```python
from build123d import *

# Parameters (mm, degrees)
F1_DEPTH = 130
F3_D     = 7
F5_D     = 5
F7_DEPTH = 25


# Not quite as in the source:
# - a feature names something its author has since deleted; it is built from what else it names


with BuildPart() as f1:
    # F0 (on Front) → F1 (new body, symmetric)
    with BuildSketch(Plane.XZ):
        Polygon((0, 30), (0, 0), (3, 0), (3, 27), (30, 27), (30, 30), align=None)
    extrude(amount=F1_DEPTH, both=True)

    # F3 (through all)
    with Locations(Plane(origin=(0, 0, 0), x_dir=(0, -1, 0), z_dir=(-1, 0, 0))):
        with Locations((-31.5, 10), (31.5, 10)):
            Hole(F3_D / 2)

    # F5 (through all)
    with Locations(Plane.XY.offset(30)):
        with Locations((14.7187495604, 0), (14.7187495604, -100), (14.7187495604, 100), (14.7187495604, -120), (14.7187495604, 120)):
            Hole(F5_D / 2)

    # F6 (on face) → F7 (cut)
    with BuildSketch(Plane(origin=(0, 0, 0), x_dir=(0, -1, 0), z_dir=(-1, 0, 0))):
        Polygon((-85, 0), (-130, 25), (-130, 0), align=None)
        Polygon((130, 0), (130, 25), (85, 0), align=None)
    extrude(amount=-F7_DEPTH, mode=Mode.SUBTRACT)


solid = f1.part
```
Design review of the part built by this model. Coordinates are the model's own, in mm. A direction names the side the tool comes from. Coordinates: 2 decimals unless noted, no trailing zeros. Order: outer loops, then holes, each group sorted by start corner. A loop starts at its lowest first (then second) coordinate and runs counter-clockwise, first axis right, second up. Notation, with made-up numbers: (9, 87.25) -> (52, 87.25) arc R5 ccw to (52, 96.25) -> close; hole circle Ø10 at (11, -2). An arc over 180 degrees is marked (long way). One line per item, written item: value. Start each with the question number.
Q1. Insertion check: pin 1 Ø8 at (y, z) = (53.5, 5.5) entering from +X; pin 2 Ø6 at (x, y) = (22.5, 19.5) entering from -Z; pin 3 Ø10 at (x, z) = (4, 19.5) entering from -Y; pin 4 Ø1 at (y, z) = (103, 18.5) entering from -X. Each pin has a flat end and moves straight along its axis. Give the tip position at first contact, or say it passes through.
Q2. Take a section at C-C, the plane y = 0. State the section outline as (x, z) points, then the cut area to 3 significant figures.
Q3. Tool access review of faces 5 (the flat face through (19, -2, 27)), 6 (the flat face through (15, -130, 29)): name each direction out of +Z, -Z, +X, -X, +Y, -Y from which nothing blocks a thin tool from reaching the whole face with its end or side.
Q4. Take a section at D-D, the plane x = 21.25. State the section outline as (y, z) points, then the cut area to 3 significant figures.
Q5. For probe 1 along Z at (x, y) = (1.55, 31.5); probe 2 along X at (y, z) = (73, 20.5); probe 3 along Z at (x, y) = (22.75, -110), list the stretches that pass through material, from the lowest coordinate up.
Q6. Take a section at B-B, the plane z = 10. State the section outline as (x, y) points.
Q7. Mouldability with a two-part tool opening along Z and no side actions: class faces 1 (the flat face through (19, -2, 30)), 2 (the flat face through (1.479, -107.815, 12.675)), 3 (the flat face through (0, -2, 15)), 4 (the cylindrical face through (1.521, 33.115, 6.895)) as pulls with the +Z half, pulls with the -Z half, needs draft (parallel to the pull), parting line crosses it, or undercut.
Q8. Take a section at A-A, the plane y = 31.5. State the section outline as (x, z) points, then the cut area to 3 significant figures.
Values follow:
1. pin 1: stops at x = 3
1. pin 2: stops at z = 27
1. pin 3: stops at y = -128.92
1. pin 4: stops at x = 0
2. outline: (0, 0) -> (3, 0) -> (3, 27) -> (12.22, 27) -> (12.22, 30) -> (0, 30) -> close; (17.22, 27) -> (30, 27) -> (30, 30) -> (17.22, 30) -> close
2. area: 156 mm2
3. face 5: -Z, +X, +Y, -Y
3. face 6: +Z, -Z, +X, -X, -Y
4. outline: (-130, 27) -> (130, 27) -> (130, 30) -> (-130, 30) -> close
4. area: 780 mm2
5. probe 1: z = 0 to 6.5, 13.5 to 30
5. probe 2: x = 0 to 3
5. probe 3: z = 27 to 30
6. outline: (0, -103) -> (3, -103) -> (3, -35) -> (0, -35) -> close; (0, -28) -> (3, -28) -> (3, 28) -> (0, 28) -> close; (0, 35) -> (3, 35) -> (3, 103) -> (0, 103) -> close
7. face 1: pulls with the +Z half
7. face 2: pulls with the -Z half
7. face 3: needs draft
7. face 4: undercut
8. outline: (0, 0) -> (3, 0) -> (3, 6.5) -> (0, 6.5) -> close; (0, 13.5) -> (3, 13.5) -> (3, 27) -> (30, 27) -> (30, 30) -> (0, 30) -> close
8. area: 150 mm2
